```python
from build123d import *

# Parameters (mm, degrees)
ESQUISSE2_W                  = 4
ESQUISSE2_H                  = 6
ENL_V_MAT_EXTRU_1_DEPTH      = 37.503424497
R_P_TITION_CIRCULAIRE1_COUNT = 4
R_P_TITION_CIRCULAIRE1_ANGLE = 135


with BuildPart() as part:
    # Esquisse1 → Base-Révolution (revolve)
    with BuildSketch(Plane.XY, mode=Mode.PRIVATE) as base_r_volution_sk:
        Polygon((0, 12), (0, 15), (0.5, 15.5), (10, 15.5), (10, 13), (7, 13), (7, 12), align=None)
    revolve(base_r_volution_sk.sketch.rotate(Axis((-2, 0, 0), (1, 0, 0)), 90), axis=Axis((-2, 0, 0), (1, 0, 0)))

    # Esquisse2 → Enlèv. mat.-Extru.1 (cut, through all)
    with BuildSketch(Plane(origin=(0, 16, 0), x_dir=(-1, 0, 0), z_dir=(0, 1, 0))):
        with Locations((-9, 0)):
            Rectangle(ESQUISSE2_W, ESQUISSE2_H)
    enl_v_mat_extru_1 = extrude(amount=-ENL_V_MAT_EXTRU_1_DEPTH, mode=Mode.SUBTRACT)

    # Répétition circulaire1: Enlèv. mat.-Extru.1 ×4 about axis
    r_p_tition_circulaire1_axis = Axis((-2, 0, 0), (1, 0, 0))
    for i in range(1, R_P_TITION_CIRCULAIRE1_COUNT):
        add(enl_v_mat_extru_1.rotate(r_p_tition_circulaire1_axis, i * R_P_TITION_CIRCULAIRE1_ANGLE / (R_P_TITION_CIRCULAIRE1_COUNT - 1)), mode=Mode.SUBTRACT)


solid = part.part
```
Model file for the job. Use its own axes, mm. A direction names the side the tool comes from. Coordinates: 2 decimals unless noted, no trailing zeros. Write each loop counter-clockwise with the first axis right and the second up, starting at its lowest first coordinate (ties: lowest second). Pieces come first, ordered by that corner, then holes. Notation, with made-up numbers: (59, 2.5) - (73, 2.5) arc R30 ccw to (73, 28.5) - close; hole circle Ø11 at (39.5, -4.5). An arc over 180 degrees is marked (long way). One line per question, with ' | ' between items. Start each with the question number.
Q1. Cut at D-D, the plane x = 5. List the corners of the cut face in (y, z).
Q2. Cut at C-C, the plane x = 8.25. Give the number of separate pieces and of enclosed holes in the cut face, then the cut area to 3 significant figures.
Q3. Drill centre lines: line 1 (Y direction, x = 5, z = 0); line 2 (Y direction, x = 1.75, z = -5.5); line 3 (Z direction, x = 3.25, y = 6.5). Where is each one in solid material? Low to high. Write a range as [from, to].
Q4. Pull direction Y, two halves, no side cores. Call faces 1 (the face through (9, 14, -3)), 2 (the face through (8.52, -7.74, 11.98)), 3 (the face through (8.52, -11.98, 7.74)): pulls with the +Y half, pulls with the -Y half, needs draft (parallel to the pull), parting line crosses it, or undercut.
Q5. Pin check, flat tips, straight feed: pin 1 (4 mm diameter, centred on x = 2.5, z = -4, fed in from +Y); pin 2 (0.8 mm diameter, centred on x = 9, z = -14, fed in from -Y); pin 3 (9.5 mm diameter, centred on y = 7, z = 3.5, fed in from +X). Stop position of each tip, or through.
Q6. Cut at A-A, the plane z = 0. List the corners of the cut face in (x, y).
Q7. 3-axis set-ups, long thin cutter, end or side, ignore diameter. For faces 4 (the face through (8.52, 7.74, 11.98)), 5 (the face through (8.521, -7.715, -11.957)), 6 (the face through (8.521, -11.957, -7.715)), 7 (the face through (7, 3, -12)), 8 (the face through (9, -3, -14)): which of +Z, -Z, +X, -X, +Y, -Y reach the whole face in a straight line?
Answer below:
1) outline: circle Ø31 at (0, 0); hole circle Ø24 at (0, 0)
2) separate pieces: 8 | enclosed holes: 0 | area: 103 mm^2
3) line 1: [-15.5, -12], [12, 15.5] | line 2: [-14.49, -10.67], [10.67, 14.49] | line 3: [-14.07, -10.09], [10.09, 14.07]
4) face 1: needs draft | face 2: pulls with the -Y half | face 3: undercut
5) pin 1: y = 15.37 | pin 2: y = -7.44 | pin 3: x = 7
6) outline: (0, -15) - (0.5, -15.5) - (7, -15.5) - (7, -12) - (0, -12) - close; (0, 12) - (7, 12) - (7, 15.5) - (0.5, 15.5) - (0, 15) - close
7) face 4: +X, +Y | face 5: +X, -Y | face 6: -Z, +X | face 7: +X | face 8: +Z, -Z, +X
